The drawing under review shows one solid part. Ordinate dimensions are in mm from its lowest x, y, z. Round coordinates to 2 decimals unless told otherwise and drop trailing zeros. Order: outer loops, then holes, each group sorted by start corner. A loop starts at its lowest first (then second) coordinate and runs counter-clockwise, first axis right, second up. Notation, with made-up numbers: M -11.75,26 L 5.25,26 A3 cw 5.25,31 Z; hole C -8,-31.5 d6. An arc over 180 degrees is marked long. Answer as a JSON object with one key per item and string values. Group by question number.
1. To check wall thickness, follow probe 1 along Z at (x, y) = (2.55, 90) (1 decimal); probe 2 along Z at (x, y) = (0.75, 52.5) (1 decimal); probe 3 along Z at (x, y) = (0.7, 52) (1 decimal). State the ranges of each line that lie inside material, in increasing order. Write a range as [from, to].
2. Clearance check with flat-ended pins moving along their axes: P1, Ø1.5, axis at x = 1.5, z = 139.5, coming from the -Y side (1 decimal); P2, Ø12, axis at y = 88.5, z = 148, coming from the -X side. State where each tip first meets the part, or that it passes through.
3. Add section A-A on z = 85. State the section outline as (x, y) points.
4. Add section C-C on x = 2.2. State the section outline as (y, z) points (1 decimal), and give its area (3 significant figures).
5. Add section B-B on y = 95. State the section outline as (x, z) points.
6. Add section D-D on z = 43.5. State the section outline as (x, y) points (1 decimal).
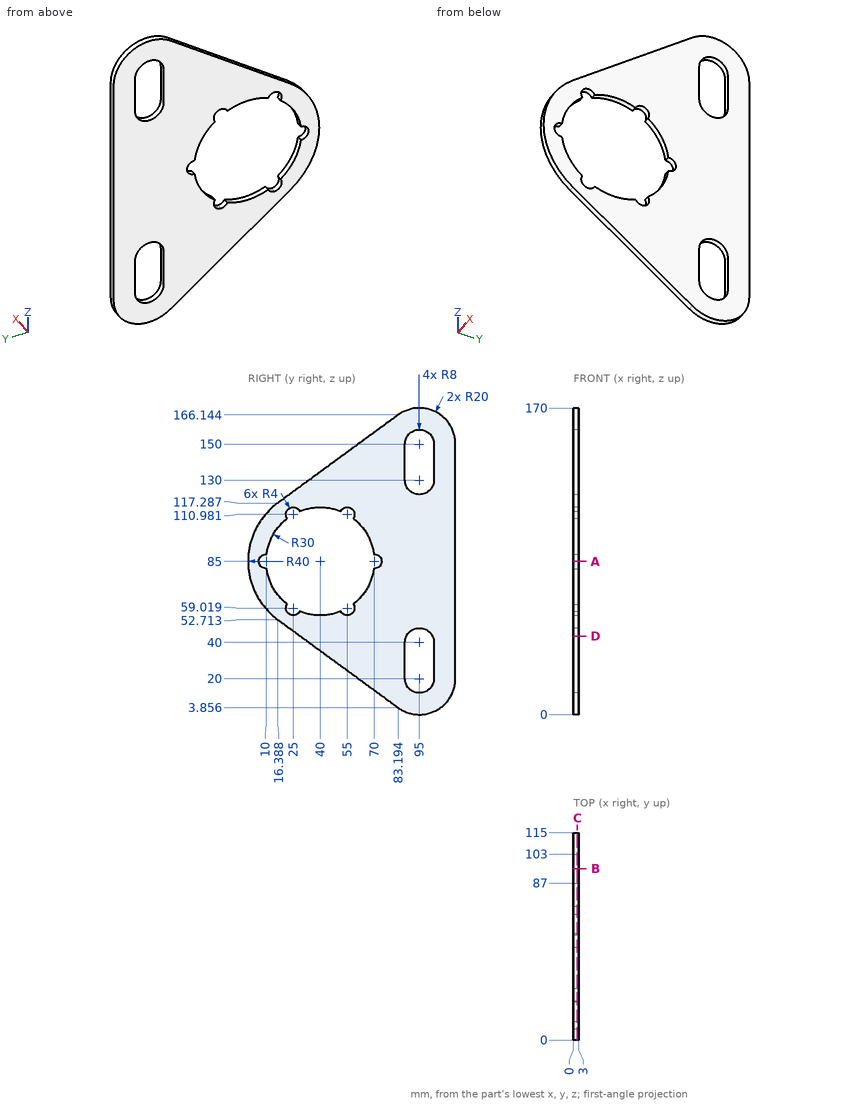
Recorded:
{
 "1": {"probe 1": "z = [0.6, 13.8], [46.2, 123.8], [156.2, 169.4]", "probe 2": "z = [26.3, 55.9], [114.1, 143.7]", "probe 3": "z = [26.7, 56.4], [113.6, 143.3]"},
 "2": {"P1": "stops at y = 45.7", "P2": "stops at x = 0"},
 "3": {"outline": "M 0,0 L 3,0 L 3,6 L 0,6 Z; M 0,74 L 3,74 L 3,115 L 0,115 Z"},
 "4": {"outline": "M 16.4,52.7 L 83.2,3.9 A20 ccw 115,20 L 115,150 A20 ccw 83.2,166.1 L 16.4,117.3 A40 ccw Z; hole M 10.3,81 A30 ccw 21.7,61.2 A4 ccw long 28.6,57.3 A30 ccw 51.4,57.3 A4 ccw long 58.3,61.2 A30 ccw 69.7,81 A4 ccw long 69.7,89 A30 ccw 58.3,108.8 A4 ccw long 51.4,112.7 A30 ccw 28.6,112.7 A4 ccw long 21.7,108.8 A30 ccw 10.3,89 A4 ccw long Z; hole M 87,20 A8 ccw 103,20 L 103,40 A8 ccw 87,40 Z; hole M 87,130 A8 ccw 103,130 L 103,150 A8 ccw 87,150 Z", "area": "9,500 mm²"},
 "5": {"outline": "M 0,0 L 3,0 L 3,12 L 0,12 Z; M 0,48 L 3,48 L 3,122 L 0,122 Z; M 0,158 L 3,158 L 3,170 L 0,170 Z"},
 "6": {"outline": "M 0,29 L 3,29 L 3,87.8 L 0,87.8 Z; M 0,102.2 L 3,102.2 L 3,115 L 0,115 Z"}
}
